from build123d import *

# Parameters (mm, degrees)
BOSS_EXTRUDE1_DEPTH = 10
SKETCH5_R           = 2
CUT_EXTRUDE1_DEPTH  = 122.881115044
FILLET3_R           = 2
FILLET4_R           = 2


with BuildPart() as part:
    # Sketch3 → Boss-Extrude1 (new body)
    with BuildSketch(Plane.XY):
        with BuildLine():
            Line((-32.260936358, 25.087487365), (-47.260936358, 21.068249478))
            Line((-47.260936358, 21.068249478), (-29.84423885, -43.931750522))
            ThreePointArc((-29.84423885, -43.931750522), (-34.146547057, -57.548288053), (-23.353857896, -66.899106783))
            Line((-23.353857896, -66.899106783), (-19.821063106, -111.899106783))
            Line((-19.821063106, -111.899106783), (-9.821063106, -111.899106783))
            Line((-9.821063106, -111.899106783), (0.506029252, -31.899106783))
            Line((0.506029252, -31.899106783), (-5.493970748, -33.506801938))
            Line((-5.493970748, -33.506801938), (-15.353857896, -46.107699741))
            Line((-15.353857896, -46.107699741), (-23.353857896, -38.289669035))
            Line((-23.353857896, -38.289669035), (-32.260936358, 25.087487365))
        make_face()
    extrude(amount=BOSS_EXTRUDE1_DEPTH)

    # Sketch5 → Cut-Extrude1 (cut, through all)
    with BuildSketch(Plane.XY.offset(10)):
        with Locations((-42.361956872, 18.239822354)):
            Circle(SKETCH5_R)
    extrude(amount=-CUT_EXTRUDE1_DEPTH, mode=Mode.SUBTRACT)

    # Fillet3
    fillet3_edges = [part.edges().sort_by_distance(p)[0] for p in [
        (-14.821063106, -111.899106783, 0),
        (-21.587460501, -89.399106783, 0),
        (-5.493970748, -33.506801938, 5),
        (0.506029252, -31.899106783, 5),
        (-9.821063106, -111.899106783, 5),
        (-47.260936358, 21.068249478, 5),
        (-32.260936358, 25.087487365, 5),
        (-21.587460501, -89.399106783, 10),
        (-14.821063106, -111.899106783, 10),
        (-4.657516927, -71.899106783, 10),
    ]]
    fillet(fillet3_edges, radius=FILLET3_R)

    # Fillet4
    # the kernel refuses this fillet: 2 mm, written as the material it takes off along each edge
    with BuildSketch(Plane(origin=(-17.971922396, -109.899106783, 2), x_dir=(0, -1, 0), z_dir=(0, 0, -1))) as fillet4_piece_1_section:
        Polygon((0, 0), (FILLET4_R, 0), (FILLET4_R, FILLET4_R * 0.924570354696), (FILLET4_R * 0.0782657346199, FILLET4_R * 0.996932532714), align=None)
    fillet4_piece_1 = extrude(amount=FILLET4_R, mode=Mode.PRIVATE)
    fillet4_piece_1 = fillet4_piece_1 - Plane(origin=(-17.971922396, -109.899106783, 2), x_dir=(0.6788719560344534, 0.7342566767214005, 0), z_dir=(0, 0, -1)) * Sphere(FILLET4_R, mode=Mode.PRIVATE)
    add(fillet4_piece_1, mode=Mode.SUBTRACT)
    with BuildSketch(Plane(origin=(-17.971922396, -109.899106783, 8), x_dir=(0, -1, 0), z_dir=(0, 0, 1))) as fillet4_piece_2_section:
        Polygon((0, 0), (FILLET4_R, 0), (FILLET4_R, -FILLET4_R * 0.924570354696), (FILLET4_R * 0.0782657346199, -FILLET4_R * 0.996932532714), align=None)
    fillet4_piece_2 = extrude(amount=FILLET4_R, mode=Mode.PRIVATE)
    fillet4_piece_2 = fillet4_piece_2 - Plane(origin=(-17.971922396, -109.899106783, 8), x_dir=(0.6788719560344534, 0.7342566767214005, 0), z_dir=(0, 0, 1)) * Sphere(FILLET4_R, mode=Mode.PRIVATE)
    add(fillet4_piece_2, mode=Mode.SUBTRACT)
    with BuildSketch(Plane(origin=(-19.821063106, -111.899106783, 2), x_dir=(1, 0, 0), z_dir=(0, 0, 1))) as fillet4_piece_3:
        with BuildLine():
            CenterArc((FILLET4_R * 0.924570354696, FILLET4_R), FILLET4_R, 184.488887052, 85.511112948)
            Line((-FILLET4_R * 0.0723621780181, FILLET4_R * 0.92173426538), (0, 0))
            Line((0, 0), (FILLET4_R * 0.924570354696, 0))
        make_face()
    extrude(amount=6, mode=Mode.SUBTRACT)


solid = part.part
Could you check a few things on this model? Use its own coordinates, in mm. A direction names the side the tool comes from. Give positions to 0.01 mm unless a question says otherwise; leave off trailing zeros. Loops run counter-clockwise (first coordinate to the right, second up) from the corner with the lowest first, then second, coordinate; pieces in that order, holes last. Notation, with made-up numbers: M -10,85 L 8,85 A14 ccw 8,98 Z; hole C 39.5,-19.5 d7. An arc over 180 degrees is marked long. Answer as a JSON object with one key per item and string values.
Q1. For P1, Ø5, axis at y = -5.5, z = 9, coming from the -X side; P2, Ø4.5, axis at x = -42.36, y = 18.24, coming from the +Z side; P3, Ø3, axis at y = 3.5, z = 1.5, coming from the -X side; P4, Ø3, axis at y = -76, z = 5, coming from the +X side, each with a flat end and sliding along its axis, tell me the tip position at first contact or that it passes through.
Values found:
{"P1": "stops at x = -40.81", "P2": "stops at z = 10", "P3": "stops at x = -42.96", "P4": "stops at x = -4.99"}
Q2. Suppose I cut it at A-A, the plane z = 5.25. List the corners of the cut face in (x, y) for me.
Values found:
{"outline": "M -46.74,19.14 L -29.84,-43.93 A13 ccw -23.35,-66.9 L -19.97,-110.06 A2 ccw -17.97,-111.9 L -11.58,-111.9 A2 ccw -9.6,-110.16 L 0.12,-34.86 A2 ccw -2.38,-32.67 L -4.85,-33.33 A2 ccw -5.91,-34.03 L -15.35,-46.11 L -23.35,-38.29 L -31.95,22.85 A2 ccw -34.44,24.5 L -45.33,21.59 A2 ccw Z; hole C -42.36,18.24 d4"}
Q3. Suppose I cut it at B-B, the plane x = -36.5. List the corners of the cut face in (y, z) for me.
Values found:
{"outline": "M -19.09,0 L 23.95,0 L 23.95,10 L -19.09,10 Z"}
Q4. For faces 4 (the flat face through (-3.6, -33, 4.9)), 5 (the flat face through (-38.4, -12, 4.9)), 6 (the cylindrical face through (-21.037, -88.732, 0.57)), which set-ups out of +Z, -Z, +X, -X, +Y, -Y let a thin tool reach every point of the face, with its end or its side?
Values found:
{"face 4": "+Z, -Z, +Y", "face 5": "+Z, -Z, -X", "face 6": "-Z, -X, -Y"}
Q5. Suppose I cut it at C-C, the plane y = 8. List the corners of the cut face in (x, z) for me, plus the area to 3 significant figures.
Values found:
{"outline": "M -43.76,0 L -29.86,0 L -29.86,10 L -43.76,10 Z", "area": "139 mm²"}
Q6. If we mould it in two halves opening along X, with no side actions, what happens to faces 1 (the cylindrical face through (-40.514, 17.474, 5.07)), 2 (the flat face through (-20, -42, 0)), 3 (the flat face through (-39.811, 23.065, 4.93))? For each: pulls with the +X half, pulls with the -X half, needs draft (parallel to the pull), parting line crosses it, or undercut.
Values found:
{"face 1": "undercut", "face 2": "needs draft", "face 3": "pulls with the -X half"}
Q7. If I drill on probe 1 along X at (y, z) = (18.5, 2); probe 2 along X at (y, z) = (12, 4.75); probe 3 along X at (y, z) = (-42, 7.75), over which ranges is the centre line in solid material (lowest first)? Write a range as [from, to].
Values found:
{"probe 1": "x = [-46.57, -44.34], [-40.38, -31.34]", "probe 2": "x = [-44.83, -30.42]", "probe 3": "x = [-30.36, -19.56], [-12.14, -0.8]"}
